from build123d import *

# Parameters (mm, degrees)
ESQUISSE2_R        = 1.8
BOSS_EXTRU_2_DEPTH = 5


with BuildPart() as part:
    # Esquisse2 → Boss.-Extru.2 (new body)
    with BuildSketch(Plane.XY):
        with BuildLine():
            Line((17.591007248, -13.591370514), (-13.915745379, 15.671652893))
            ThreePointArc((-13.915745379, 15.671652893), (-14.736105314, 13.582929731), (-16.758645601, 12.610774569))
            Line((-16.758645601, 12.610774569), (14.748107026, -16.652248837))
            ThreePointArc((14.748107026, -16.652248837), (17.699996299, -16.543259786), (17.591007248, -13.591370514))
        make_face()
        with BuildLine():
            Line((-16.758645601, 12.610774569), (-20.0542154, 15.671652893))
            ThreePointArc((-20.0542154, 15.671652893), (-19.073703551, 13.422777818), (-16.758645601, 12.610774569))
        make_face()
        with BuildLine():
            ThreePointArc((-16.758645601, 12.610774569), (-14.736105314, 13.582929731), (-13.915745379, 15.671652893))
            ThreePointArc((-13.915745379, 15.671652893), (-16.984980389, 18.740887903), (-20.0542154, 15.671652893))
            Line((-20.0542154, 15.671652893), (-16.758645601, 12.610774569))
        make_face()
        with Locations((-16.984980389, 15.671652893)):
            Circle(ESQUISSE2_R, mode=Mode.SUBTRACT)
    extrude(amount=BOSS_EXTRU_2_DEPTH)


solid = part.part
Here's how the part is built. I have some questions about the finished solid (model axes, mm). Give positions to 0.01 mm unless a question says otherwise; leave off trailing zeros. Order: outer loops, then holes, each group sorted by start corner. A loop starts at its lowest first (then second) coordinate and runs counter-clockwise, first axis right, second up. Notation, with made-up numbers: (25.25, -3.75) -> (73.25, -3.75) arc R12 ccw to (73.25, 12.25) -> close; hole circle Ø4 at (30, 61). An arc over 180 degrees is marked (long way). Use a Markdown table: item, result. Add a question column.
Item 1: If we mould it in two halves opening along Y, with no side actions, what happens to faces 1 (the face through (-17.219, 17.456, 2.465)), 2 (the face through (17.668, -16.577, 2.465)), 3 (the face through (-1, 0, 5))? For each: pulls with the +Y half, pulls with the -Y half, needs draft (parallel to the pull), parting line crosses it, or undercut.
Item 2: Will these pins go through, and if not, where does the flat tip stop? pin 1 (5 mm diameter, centred on x = -6, y = -1.5, fed in from +Z); pin 2 (3 mm diameter, centred on y = -12, z = 3, fed in from +X); pin 3 (1 mm diameter, centred on y = 9.5, z = 4, fed in from +X); pin 4 (2 mm diameter, centred on x = -7.5, z = 1.5, fed in from +Y).
Item 3: Imagine slicing it at C-C on y = 9.5. Please give me the cut outline in (x, z), plus the area to 3 significant figures.
Item 4: Imagine slicing it at A-A on z = 2.8. Please give me the cut outline in (x, y).
Item 5: I need wall thicknesses on line 1 (Y direction, x = -17, z = 0.4); line 2 (Y direction, x = -18, z = 1.4); line 3 (Y direction, x = -3, z = 4.85). Which ranges of each line are inside material? Lowest first, please.
Item 6: Imagine slicing it at B-B on x = 2. Please give me the cut outline in (y, z), plus the area to 3 significant figures.
Data:
| question | item | result |
|---|---|---|
| 1 | face 1 | undercut |
| 1 | face 2 | parting line crosses it |
| 1 | face 3 | needs draft |
| 2 | pin 1 | passes through |
| 2 | pin 2 | stops at x = 17.49 |
| 2 | pin 3 | stops at x = -6.73 |
| 2 | pin 4 | stops at y = 10.64 |
| 3 | outline | (-13.41, 0) -> (-7.27, 0) -> (-7.27, 5) -> (-13.41, 5) -> close |
| 3 | area | 30.7 mm² |
| 4 | outline | (-16.76, 12.61) -> (14.75, -16.65) arc R2.09 ccw to (17.59, -13.59) -> (-13.92, 15.67) arc R3.07 ccw (long way) to start; hole circle Ø3.6 at (-16.98, 15.67) |
| 5 | line 1 | y = 12.6 to 13.87, 17.47 to 18.74 |
| 5 | line 2 | y = 12.78 to 14.19, 17.16 to 18.57 |
| 5 | line 3 | y = -0.17 to 5.53 |
| 6 | outline | (-4.81, 0) -> (0.89, 0) -> (0.89, 5) -> (-4.81, 5) -> close |
| 6 | area | 28.5 mm² |
